The model under review builds one solid part; all positions refer to its coordinate system, in mm. A direction names the side the tool comes from. Round coordinates to 2 decimals unless told otherwise and drop trailing zeros. Write each loop counter-clockwise with the first axis right and the second up, starting at its lowest first coordinate (ties: lowest second). Pieces come first, ordered by that corner, then holes. Notation, with made-up numbers: (-40, 89.25) - (-31, 89.25) arc R20 cw to (-31, 116.25) - close; hole circle Ø1 at (-19.75, 84). An arc over 180 degrees is marked (long way). Write each question's results on one line, items separated by ' | '.
Autodesk Inventor part; units mm, degrees
ref_plane "YZ Plane" through (0, 0, 0) normal (1, 0, 0) x (0, 1, 0)
ref_plane "XZ Plane" through (0, 0, 0) normal (0, 1, 0) x (-1, 0, 0)
ref_plane "XY Plane" through (0, 0, 0) normal (0, 0, 1) x (1, 0, 0)
sketch "Sketch1" plane through (0, 0, 0) normal (0, 1, 0) x (-1, 0, 0)
  line L0 (16.5, 20) -> (-16.5, 20)
  line L1 (-18.5, 18) -> (-18.5, -18)
  line L2 (-16.5, -20) -> (16.5, -20)
  line L3 (18.5, -18) -> (18.5, 18)
  arc A0 (18.5, 18) -> (16.5, 20) centre (16.5, 18) ccw
  arc A1 (16.5, -20) -> (18.5, -18) centre (16.5, -18) ccw
  arc A2 (-16.5, 20) -> (-18.5, 18) centre (-16.5, 18) ccw
  arc A3 (-18.5, -18) -> (-16.5, -20) centre (-16.5, -18) ccw
  line L4 (6.5, 24) -> (-6.5, 24)
  line L5 (-7.5, 23) -> (-7.5, 20)
  line L6 (-7.5, 20) -> (7.5, 20)
  line L7 (7.5, 20) -> (7.5, 23)
  line L8 (7.5, -20) -> (-7.5, -20)
  line L9 (-7.5, -20) -> (-7.5, -23)
  line L10 (-6.5, -24) -> (6.5, -24)
  line L11 (7.5, -23) -> (7.5, -20)
  arc A4 (7.5, 23) -> (6.5, 24) centre (6.5, 23) ccw
  arc A5 (-6.5, 24) -> (-7.5, 23) centre (-6.5, 23) ccw
  arc A6 (-7.5, -23) -> (-6.5, -24) centre (-6.5, -23) ccw
  arc A7 (6.5, -24) -> (7.5, -23) centre (6.5, -23) ccw
  circle A8 centre (3, 24) radius 1.5
  circle A9 centre (-3, 24) radius 1.5
  circle A10 centre (15.25, 15.25) radius 2
  circle A11 centre (15.25, -15.25) radius 2
  circle A12 centre (-15.25, -15.25) radius 2
  circle A13 centre (-15.25, 15.25) radius 2
  point P0 (0, 0)
  point P1 (-18.5, -20)
  point P2 (-18.5, 20)
  point P3 (18.5, -20)
  point P4 (-7.5, 24)
  point P5 (-7.5, -24)
  point P6 (7.5, -24)
  point P7 (0, 20)
  point P8 (0, -20)
  point P9 (4.5, 24)
  point P10 (1.5, 24)
  point P11 (-1.5, 24)
  point P12 (-4.5, 24)
  dimension "d0" = 37
  dimension "d1" = 40
  dimension "d2" = 20
  dimension "d3" = 18.5
  dimension "d4" = 2
  dimension "d5" = 15
  dimension "d6" = 4
  dimension "d7" = 15
  dimension "d8" = 4
  dimension "d9" = 1
  dimension "d10" = 3
  dimension "d11" = 3
  dimension "d12" = 3
  dimension "d13" = 6
  dimension "d14" = 4
  dimension "d15" = 4
  dimension "d16" = 4
  dimension "d17" = 4
  dimension "d18" = 30.5
  dimension "d19" = 30.5
  dimension "d20" = 30.5
  dimension "d21" = 30.5
  dimension "d22" = 3.25
  dimension "d23" = 4.75
extrude "Extrusion1" add sketch "Sketch1" along normal blind 6 contours A0 L3 A1 L2 A3 L1 A2 L0 | L0 L5 A5 L4 A9 A8 A4 L7 | L11 A7 L10 A6 L9 L2
equation "\"d22\" = -0.5 * d20 + 0.5 * d0"
equation "\"d23\" = -0.5 * d19 + 0.5 * d1"
properties part number "Holybro Tekko ESC model" material "PMMA Plastic"
Q1. We need section C-C (x = -16). State the section outline as (y, z) points, plus the area to 3 significant figures.
Evaluation:
outline: (0, -20) - (6, -20) - (6, -17.1) - (0, -17.1) - close; (0, -13.4) - (6, -13.4) - (6, 13.4) - (0, 13.4) - close; (0, 17.1) - (6, 17.1) - (6, 20) - (0, 20) - close | area: 196 mm^2
Q2. We need section D-D (x = -3). State the section outline as (y, z) points, plus the area to 3 significant figures.
Evaluation:
outline: (0, -24) - (6, -24) - (6, 22.5) - (0, 22.5) - close | area: 279 mm^2
Q3. For probe 1 along Z at (x, y) = (15.25, 1.7); probe 2 along Z at (x, y) = (-16, 4.4); probe 3 along Z at (x, y) = (-10, 4.5), list the stretches that pass through material, from the lowest coordinate up.
Evaluation:
probe 1: z = -20 to -17.25, -13.25 to 13.25, 17.25 to 20 | probe 2: z = -20 to -17.1, -13.4 to 13.4, 17.1 to 20 | probe 3: z = -20 to 20
Q4. The part is to be moulded in two halves that separate along Z. For faces 3 (the flat face through (0, 3, 24)), 4 (the cylindrical face through (-14.99, 2.958, -17.233)), 5 (the flat face through (-7.5, 3, 21)), say which applies: released by +Z, released by -Z, zero draft, split by the parting line, or undercut.
Evaluation:
face 3: released by +Z | face 4: undercut | face 5: zero draft
Q5. We need section B-B (z = -15.25). State the section outline as (x, y) points, plus the area to 3 significant figures.
Evaluation:
outline: (-18.5, 0) - (-17.25, 0) - (-17.25, 6) - (-18.5, 6) - close; (-13.25, 0) - (13.25, 0) - (13.25, 6) - (-13.25, 6) - close; (17.25, 0) - (18.5, 0) - (18.5, 6) - (17.25, 6) - close | area: 174 mm^2
Q6. Tool access review of faces 1 (the flat face through (-6, 3, 24)), 2 (the flat face through (-12, 3, 20)): name each direction out of +Z, -Z, +X, -X, +Y, -Y from which nothing blocks a thin tool from reaching the whole face with its end or side.
Evaluation:
face 1: +Z, +X, -X, +Y, -Y | face 2: +Z, -X, +Y, -Y
Q7. We need section A-A (y = 1.1). State the section outline as (x, z) points.
Evaluation:
outline: (-18.5, -18) arc R2 ccw to (-16.5, -20) - (-7.5, -20) - (-7.5, -23) arc R1 ccw to (-6.5, -24) - (6.5, -24) arc R1 ccw to (7.5, -23) - (7.5, -20) - (16.5, -20) arc R2 ccw to (18.5, -18) - (18.5, 18) arc R2 ccw to (16.5, 20) - (7.5, 20) - (7.5, 23) arc R1 ccw to (6.5, 24) - (4.5, 24) arc R1.5 cw to (1.5, 24) - (-1.5, 24) arc R1.5 cw to (-4.5, 24) - (-6.5, 24) arc R1 ccw to (-7.5, 23) - (-7.5, 20) - (-16.5, 20) arc R2 ccw to (-18.5, 18) - close; hole circle Ø4 at (-15.25, -15.25); hole circle Ø4 at (-15.25, 15.25); hole circle Ø4 at (15.25, -15.25); hole circle Ø4 at (15.25, 15.25)
Q8. Insertion check: P1, Ø1.5, axis at y = 4, z = -21.5, coming from the -X side; P2, Ø1.8, axis at x = 13, y = 2, coming from the -Z side; P3, Ø2.5, axis at x = -15.25, z = 15.25, coming from the +Y side; P4, Ø3.5, axis at y = 2, z = 21.5, coming from the -X side. Each pin has a flat end and moves straight along its axis. Give the tip position at first contact, or say it passes through.
Evaluation:
P1: stops at x = -7.5 | P2: stops at z = -20 | P3: passes through | P4: stops at x = -17.47
